Autodesk Fusion 360 part; units mm, degrees
sketch "Sketch1" plane through (0, 0, 0) normal (0, 0, 1) x (1, 0, 0)
  line L0 (51, 42) -> (0, 42)
  line L1 (0, 42) -> (0, 0)
  line L2 (0, 0) -> (54, 0)
  line L3 (54, 0) -> (66, 12)
  line L4 (66, 12) -> (66, 27)
  line L5 (66, 27) -> (51, 42)
extrude "Extrude1" add sketch "Sketch1" along normal blind 12 makes body 1
sketch "Sketch2" plane through (0, 0, 0) normal (0, 0, 1) x (1, 0, 0)
  line L0 (0, 0) -> (12, 0)
  line L1 (12, 0) -> (12, 42)
  line L2 (12, 42) -> (0, 42)
  line L3 (0, 42) -> (0, 0)
extrude "Extrude2" add sketch "Sketch2" along normal blind 39 bodies 1
sketch "Sketch3" plane through (0, 0, 0) normal (1, 0, 0) x (0, 1, 0)
  line L0 (42, 39) -> (0, 39)
  arc A0 (42, 39) -> (0, 39) centre (21, 39) ccw
extrude "Extrude3" add sketch "Sketch3" along normal blind 12 bodies 1
sketch "Sketch4" plane through (0, 0, 0) normal (0, 1, 0) x (1, 0, 0)
  line L0 (12, -12) -> (12, -54)
  line L1 (12, -54) -> (66, -12)
  line L2 (66, -12) -> (12, -12)
extrude "Extrude4" add sketch "Sketch4" along normal blind 12 separate body makes body 2
move_body "Move1" bodies 2 to x (1, 0, 0) y (0, 1, 0) z (0, 0, 1) at (0, 15, 0)
combine "Combine1" operation add target body 1 tool bodies 2
The listing builds one solid part. Answer for the finished solid, in the listing's coordinates (mm). A direction names the side the tool comes from. Coordinates: 2 decimals unless noted, no trailing zeros. Order: outer loops, then holes, each group sorted by start corner. A loop starts at its lowest first (then second) coordinate and runs counter-clockwise, first axis right, second up.
Q1. A cutting plane is placed at D-D, the plane y = 13. Write down the section's boundary in (x, z).
Q2. A cutting plane is placed at C-C, the plane x = 27.5. Write down the section's boundary in (y, z), and give its area (3 significant figures).
Q3. A cutting plane is placed at A-A, the plane z = 26. Write down the section's boundary in (x, y).
Q4. Consider line 1 (X direction, y = 10, z = 26.5); line 2 (Y direction, x = 23, z = 31). Determine where each line is inside the solid, lowest interval first.
Q5. Given P1, Ø4.5, axis at x = 51, y = 9, coming from the +Z side; P2, Ø4, axis at y = 37, z = 52, coming from the +X side; P3, Ø5, axis at x = 31.5, y = 21.5, coming from the +Z side; P4, Ø12.5, axis at x = 44, z = 42, coming from the +Y side, each flat-ended and moving along its own axis, determine where each tip first touches the part or whether it passes through.
Q6. Which of the six approach directions +Z, -Z, +X, -X, +Y, -Y give full straight-line access (tool end or side, diameter ignored) to faces 1 (the face through (12, 30, 36)), 2 (the face through (33, 27, 28)), 3 (the face through (39, 21, 33)), 4 (the face through (39, 8, 12))?
Q7. A cutting plane is placed at B-B, the plane y = 21. Write down the section's boundary in (x, z), and give its area (3 significant figures).
Answers follow:
1. outline: (0, 0) - (66, 0) - (66, 12) - (12, 12) - (12, 58.42) - (0, 58.42) - close
2. outline: (0, 0) - (42, 0) - (42, 12) - (27, 12) - (27, 41.94) - (15, 41.94) - (15, 12) - (0, 12) - close
2. area: 863 mm2
3. outline: (0, 0) - (12, 0) - (12, 15) - (48, 15) - (48, 27) - (12, 27) - (12, 42) - (0, 42) - close
4. line 1: x = 0 to 12
4. line 2: y = 15 to 27
5. P1: stops at z = 12
5. P2: stops at x = 12
5. P3: stops at z = 40.78
5. P4: passes through
6. face 1: +Z, +X
6. face 2: +Z, +X, +Y
6. face 3: +Z, +X, +Y, -Y
6. face 4: +Z, +X, -Y
7. outline: (0, 0) - (66, 0) - (66, 12) - (12, 54) - (12, 60) - (0, 60) - close
7. area: 2,500 mm2
